Check sheet for the modelled part. Datum: model origin and axes. Units: mm. A direction names the side the tool comes from. Round coordinates to 2 decimals unless told otherwise and drop trailing zeros. Order: outer loops, then holes, each group sorted by start corner. A loop starts at its lowest first (then second) coordinate and runs counter-clockwise, first axis right, second up.
(1) Tool access check on faces 1 (the flat face through (0, 0, 3.4)), 2 (the cylindrical face through (-1.5, 0.07, 2.64)). Record the directions out of +Z, -Z, +X, -X, +Y, -Y that give a thin tool (end or side, any length) a straight path to the whole face; none if there is none.
(2) Sectioned sample at D-D, the plane x = -2. Enter the section's corners in (y, z), and give its area (3 significant figures).
(3) Thickness scan on probe 1 along Z at (x, y) = (0.5, -2.75); probe 2 along X at (y, z) = (-1, 2.55); probe 3 along X at (y, z) = (-1.25, 1.55). Record the ranges inside material, lowest first.
(4) Sectioned sample at B-B, the plane y = 0. Enter the section's corners in (x, z).
(5) Sectioned sample at C-C, the plane z = 2.8. Enter the section's corners in (x, y), and give its area (3 significant figures).
(6) Sectioned sample at A-A, the plane x = 0. Enter the section's corners in (y, z).
(7) Depth check by flat-ended pin: pin 1 (1.5 mm diameter, centred on x = 5.5, y = -1, fed in from +Z); pin 2 (5 mm diameter, centred on x = -1, y = 2, fed in from +Z). Enter the tip coordinate at first touch or a pass-through.
```python
from build123d import *

# Parameters (mm, degrees)
PAD_DEPTH    = 0.5
SKETCH_R     = 1.5
PAD001_DEPTH = 1.5


with BuildPart() as part:
    # Sketch002 → Pad (new body)
    with BuildSketch(Plane.XY.offset(1.4)):
        with BuildLine():
            ThreePointArc((-2.5, 5), (-7.5, 0), (-2.5, -5))
            Line((-2.5, -5), (2.5, -5))
            ThreePointArc((2.5, -5), (7.5, 0), (2.5, 5))
            Line((-2.5, 5), (2.5, 5))
        make_face()
    extrude(amount=PAD_DEPTH)

    # Sketch (on Face6 of Pad) → Pad001 (join)
    with BuildSketch(Plane.XY.offset(1.9)):
        Circle(SKETCH_R)
    extrude(amount=PAD001_DEPTH)


solid = part.part
```
Derived:
1. face 1: +Z, +X, -X, +Y, -Y
1. face 2: +Z
2. outline: (-5, 1.4) - (5, 1.4) - (5, 1.9) - (-5, 1.9) - close
2. area: 5.00 mm2
3. probe 1: z = 1.4 to 1.9
3. probe 2: x = -1.12 to 1.12
3. probe 3: x = -7.34 to 7.34
4. outline: (-7.5, 1.4) - (7.5, 1.4) - (7.5, 1.9) - (1.5, 1.9) - (1.5, 3.4) - (-1.5, 3.4) - (-1.5, 1.9) - (-7.5, 1.9) - close
5. outline: circle Ø3 at (0, 0)
5. area: 7.07 mm2
6. outline: (-5, 1.4) - (5, 1.4) - (5, 1.9) - (1.5, 1.9) - (1.5, 3.4) - (-1.5, 3.4) - (-1.5, 1.9) - (-5, 1.9) - close
7. pin 1: stops at z = 1.9
7. pin 2: stops at z = 3.4
